Build history of the part. All positions in model axes, mm. A direction names the side the tool comes from. Give positions to 0.01 mm unless a question says otherwise; leave off trailing zeros. Order: outer loops, then holes, each group sorted by start corner. A loop starts at its lowest first (then second) coordinate and runs counter-clockwise, first axis right, second up. Notation, with made-up numbers: (84.5, 20) -> (143.5, 20) arc R20 ccw to (143.5, 56) -> close; hole circle Ø5 at (11, 75). An arc over 180 degrees is marked (long way). One line per item, written item: value. Start each with the question number.
(1) Saw through at C-C on z = -3. Give the cut face in (x, y), plus the area to 3 significant figures.
(2) Saw through at A-A on x = -15. Give the cut face in (y, z), plus the area to 3 significant figures.
(3) Two-plate mould, pull along X, no slides. Class faces 5 (the flat face through (-15, 40, -17.25)), 6 (the flat face through (-26, 12, -15)), 7 (the cylindrical face through (-13.8, 42.555, -14.968)): +X half, -X half, draft (parallel to the pull), parting line (faces both ways), or undercut.
(4) Which spindle directions (+Z, -Z, +X, -X, +Y, -Y) get a long thin tool onto all of the face, cutting with end or side? Do faces 1 (the flat face through (-15, 50, -15)), 2 (the flat face through (-20, 40, -15)), 3 (the flat face through (-10, 40, -15)), 4 (the flat face through (-15, 40, -12.75)). Say none if no direction does.
(5) Saw through at B-B on y = 32. Give the cut face in (x, z), plus the area to 3 significant figures.
(6) Probe line 1 (Y direction, x = -15, z = -14.4); line 2 (Z direction, x = -18, y = 45.5); line 3 (Z direction, x = -5.5, y = 6). List the from-to ranges inside material, lowest first.
(7) Pin check, flat tips, straight feed: pin 1 (3 mm diameter, centred on x = -15, y = 44.86, fed in from +Z); pin 2 (2 mm diameter, centred on y = 38.5, z = -14, fed in from -X); pin 3 (5 mm diameter, centred on x = -26, y = 7, fed in from -Z); pin 4 (8 mm diameter, centred on x = -15.5, y = 38.5, fed in from +Z). Stop position of each tip, or through.
Autodesk Inventor part; units mm, degrees
ref_plane "YZ Plane" through (0, 0, 0) normal (1, 0, 0) x (0, 1, 0)
ref_plane "XZ Plane" through (0, 0, 0) normal (0, 1, 0) x (-1, 0, 0)
ref_plane "XY Plane" through (0, 0, 0) normal (0, 0, 1) x (1, 0, 0)
sketch "Sketch1" plane through (0, 0, 0) normal (0, 1, 0) x (-1, 0, 0)
  line L0 (0, 0) -> (30, 0)
  line L1 (30, 0) -> (30, -30)
  line L2 (30, -30) -> (0, -30)
  line L3 (0, -30) -> (0, 0)
  dimension "d0" = 30
  dimension "d1" = 30
extrude "Extrusion1" add sketch "Sketch1" along normal blind 30
sketch "Sketch2" plane through (0, 30, 0) normal (0, 1, 0) x (1, 0, 0)
  line L0 (-20, 17.25) -> (-10, 17.25)
  line L1 (-10, 17.25) -> (-10, 12.75)
  line L2 (-10, 12.75) -> (-20, 12.75)
  line L3 (-20, 12.75) -> (-20, 17.25)
  line L4 (-20, 17.25) -> (-10, 12.75) construction
  line L5 (-10, 17.25) -> (-20, 12.75) construction
  line L6 (-30, 30) -> (-30, 0)
  line L7 (-30, 0) -> (0, 0)
  point P0 (-15, 15)
  point P1 (-30, 15)
  dimension "d4" = 15
  dimension "d5" = 15
  dimension "d6" = 10
  dimension "d7" = 4.5
extrude "Extrusion2" add sketch "Sketch2" along normal blind 20
sketch "Sketch3" plane through (-20, 30, -12.75) normal (0, 0, 1) x (1, 0, 0)
  circle A0 centre (5, 14.8617) radius 2.6
  point P0 (20, -30)
  dimension "d10" = 5.2
extrude "Extrusion3" cut sketch "Sketch3" against normal blind 20
sketch "Sketch4" plane through (-30, 0, 0) normal (0, 0, 1) x (1, 0, 0)
  line L0 (10, 30) -> (20, 30)
  line L1 (0, 0) -> (0, 30)
  line L2 (10, 30) -> (0, 0)
  line L3 (0, 0) -> (0, 30)
  line L4 (0, 30) -> (10, 30)
  line L5 (0, 30) -> (30, 30)
  line L6 (20.2474, 30) -> (30, 0)
  line L7 (30, 0) -> (30, 30)
  line L8 (30, 0) -> (30, 30)
  line L9 (30, 30) -> (20.2474, 30)
extrude "Extrusion4" cut sketch "Sketch4" against normal blind 71.25
sketch "Sketch6" plane through (-10, 30, -12.75) normal (1, 0, 0) x (0, 0, -1)
  line L0 (0, 0) -> (-12.75, -30)
  line L1 (-12.75, -30) -> (-12.75, 0)
  line L2 (-12.75, -30) -> (-12.75, 0)
  line L3 (0, 0) -> (-12.75, 0)
  line L4 (-12.75, 0) -> (0, 0)
  line L5 (17.25, 0) -> (4.5, 0)
  line L6 (0, 0) -> (4.5, 0)
  line L7 (4.5, 0) -> (17.25, 0)
  line L8 (17.25, 0) -> (17.25, -30)
  line L9 (17.25, 0) -> (17.25, -30)
  line L10 (4.5, 0) -> (4.5, 20)
  line L11 (17.25, -30) -> (4.5, 0)
extrude "Extrusion5" cut sketch "Sketch6" along normal blind 71.25 and the other way blind 35.625
properties part number "ObjectPyrsmid"
Results below:
1. outline: (-30, 0) -> (0, 0) -> (-2.29, 7.06) -> (-27.65, 7.06) -> close
1. area: 195 mm²
2. outline: (0, -30) -> (30, -17.25) -> (42.26, -17.25) -> (42.26, -12.75) -> (30, -12.75) -> (0, 0) -> close; (47.46, -17.25) -> (50, -17.25) -> (50, -12.75) -> (47.46, -12.75) -> close
2. area: 584 mm²
3. face 5: draft
3. face 6: -X half
3. face 7: undercut
4. face 1: +Z, -Z, +X, -X, +Y
4. face 2: +Z, -Z, -X, +Y
4. face 3: +Z, -Z, +X, +Y
4. face 4: +Z, +X, -X, +Y
5. outline: (-20, -17.25) -> (-10, -17.25) -> (-10, -12.75) -> (-20, -12.75) -> close
5. area: 45.0 mm²
6. line 1: y = 0 to 42.26, 47.46 to 50
6. line 2: z = -17.25 to -12.75
6. line 3: z = -27.45 to -2.55
7. pin 1: passes through
7. pin 2: stops at x = -20
7. pin 3: stops at z = -28.09
7. pin 4: stops at z = -12.75
